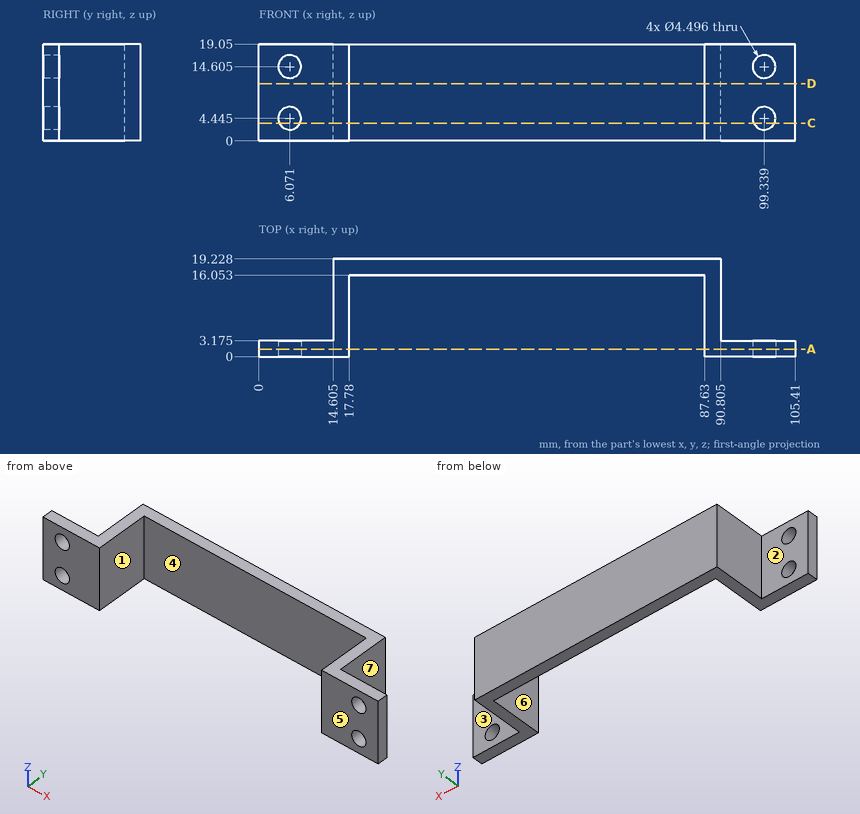
Can you work these out from the drawing? Everything is in mm from the part's minimum corner. A direction names the side the tool comes from. Coordinates: 2 decimals unless noted, no trailing zeros. Write each loop counter-clockwise with the first axis right and the second up, starting at its lowest first coordinate (ties: lowest second). Pieces come first, ordered by that corner, then holes. Notation, with made-up numbers: (-25.5, 21.25) -> (-1.5, 21.25) arc R21 cw to (-1.5, 29.25) -> close; hole circle Ø5 at (15, -31). An arc over 180 degrees is marked (long way). Write item = value, one per line.
(1) Imagine slicing it at A-A (y = 1.5). State how many separate pieces and enclosed holes the cut face has, and give its area (3 significant figures).
Verdict:
separate_pieces = 2
enclosed_holes = 4
area = 614 mm^2
(2) Thinking about a two-plate mould opening in X: for the marked faces 4, 5, 6 and 7, which applies, +X half, -X half, draft (parallel to the pull), parting line (faces both ways), or undercut?
Verdict:
face_4 = undercut
face_5 = draft
face_6 = undercut
face_7 = +X half
(3) If I drill on probe 1 along X at (y, z) = (1.75, 4.75); probe 2 along X at (y, z) = (7.5, 17.75) (1 decimal); probe 3 along Y at (x, z) = (20, 5.25), over which ranges is the centre line in solid material (lowest first)?
Verdict:
probe_1 = 0 to 3.84, 8.3 to 17.78, 87.63 to 97.11, 101.57 to 105.41
probe_2 = 14.6 to 17.8, 87.6 to 90.8
probe_3 = 16.05 to 19.23
(4) For pin 1 (8 mm diameter, centred on y = 7.5, z = 10, fed in from -X) (3 decimals); pin 2 (2 mm diameter, centred on x = 22, z = 13, fed in from -Y); pin 3 (3 mm diameter, centred on y = 4, z = 5.5, fed in from +X); pin 4 (2.5 mm diameter, centred on x = 99.34, z = 14.6, fed in from -Y), each with a flat end and sliding along its axis, tell me the tip position at first contact or that it passes through.
Verdict:
pin_1 = 14.605
pin_2 = 16.05
pin_3 = 105.41
pin_4 = through
(5) Imagine slicing it at C-C (z = 3.5). Please give me the cut outline in (x, y) (1 decimal).
Verdict:
outline = (0, 0) -> (4, 0) -> (4, 3.2) -> (0, 3.2) -> close; (8.1, 0) -> (17.8, 0) -> (17.8, 16.1) -> (87.6, 16.1) -> (87.6, 0) -> (97.3, 0) -> (97.3, 3.2) -> (90.8, 3.2) -> (90.8, 19.2) -> (14.6, 19.2) -> (14.6, 3.2) -> (8.1, 3.2) -> close; (101.4, 0) -> (105.4, 0) -> (105.4, 3.2) -> (101.4, 3.2) -> close
(6) On a 3-axis mill with a long thin cutter (end or side, diameter ignored), from which of +Z, -Z, +X, -X, +Y, -Y can I reach the whole of each face in a straight line? I mean the marked faces 1, 2 and 3. Say none if no direction works.
Verdict:
face_1 = +Z, -Z, -Y
face_2 = +Z, -Z, -X, +Y
face_3 = +Z, -Z, +X, +Y
(7) Imagine slicing it at D-D (z = 11.25). Please give me the cut outline in (x, y) (1 decimal).
Verdict:
outline = (0, 0) -> (17.8, 0) -> (17.8, 16.1) -> (87.6, 16.1) -> (87.6, 0) -> (105.4, 0) -> (105.4, 3.2) -> (90.8, 3.2) -> (90.8, 19.2) -> (14.6, 19.2) -> (14.6, 3.2) -> (0, 3.2) -> close
